For this review, take the finished solid that the model builds, in its own axes (mm). Coordinates: 2 decimals unless noted, no trailing zeros. Write each loop counter-clockwise with the first axis right and the second up, starting at its lowest first coordinate (ties: lowest second). Pieces come first, ordered by that corner, then holes.
1) Mouldability with a two-part tool opening along Y and no side actions: class faces 1 (the face through (1.972, -0.717, 4.943)), 2 (the face through (2.028, -0.09, -3.024)), 3 (the face through (4, 0, 2)) as pulls with the +Y half, pulls with the -Y half, needs draft (parallel to the pull), parting line crosses it, or undercut.
2) To check wall thickness, follow line 1 along Z through (x, y) = (0.85, 4.75); line 2 along Z through (x, y) = (2.9, 0) (3 decimals); line 3 along Y through (x, z) = (1.7, 0) (3 decimals). State the ranges of each line that lie inside material, in increasing order.
3) Insertion check: P1, Ø6, axis at y = -3.5, z = -3, coming from the -X side; P2, Ø1, axis at x = 2.5, y = 4, coming from the +Z side. Each pin has a flat end and moves straight along its axis. Give the tip position at first contact, or say it passes through.
4) We need section D-D on z = -4.5. Write out the cut boundary in (x, y).
5) We need section A-A on z = 0. Write out the cut boundary in (x, y) (3 decimals), then the cut area to 3 significant figures.
6) We need section B-B on y = -1.5. Write out the cut boundary in (x, z) (3 decimals).
7) We need section C-C on z = 4. Write out the cut boundary in (x, y).
from build123d import *

# Parameters (mm, degrees)
BASPROSKE_W         = 4
BASPROSKE_H         = 6
TOOTHCUT_DEPTH      = 10.38083152
TEETHCUTS_COUNT     = 10
TEETHCUTS_ANGLE     = 324
BORSKE_R            = 3.025
BORE_DEPTH          = 50.0000508
BOSS_EXTRUDE1_DEPTH = 4


with BuildPart() as part:
    # BasProSke → Base-Revolve (revolve)
    with BuildSketch(Plane(origin=(0, 0, 0), x_dir=(1, 0, 0), z_dir=(0, 1, 0)), mode=Mode.PRIVATE) as base_revolve_sk:
        with Locations((2, 3)):
            Rectangle(BASPROSKE_W, BASPROSKE_H)
    revolve(base_revolve_sk.sketch.rotate(Axis((-10, 0, 0), (1, 0, 0)), 180), axis=Axis((-10, 0, 0), (1, 0, 0)))

    # TooCutSke → ToothCut (cut, through all)
    with BuildSketch(Plane(origin=(0, 0, 0), x_dir=(0, 0, -1), z_dir=(1, 0, 0))):
        with BuildLine():
            ThreePointArc((0.59278292, 3.701838653), (0, 3.749), (-0.59278292, 3.701838653))
            ThreePointArc((-0.59278292, 3.701838653), (-0.846593509, 4.924114224), (-1.775771316, 5.757784417))
            ThreePointArc((-1.775771316, 5.757784417), (0, 6.0254), (1.775771316, 5.757784417))
            ThreePointArc((1.775771316, 5.757784417), (0.846593509, 4.924114224), (0.59278292, 3.701838653))
        make_face()
    toothcut = extrude(amount=TOOTHCUT_DEPTH, mode=Mode.SUBTRACT)

    # TeethCuts: ToothCut ×10 about axis
    teethcuts_axis = Axis((-10, 0, 0), (1, 0, 0))
    for i in range(1, TEETHCUTS_COUNT):
        add(toothcut.rotate(teethcuts_axis, i * TEETHCUTS_ANGLE / (TEETHCUTS_COUNT - 1)), mode=Mode.SUBTRACT)

    # BorSke → Bore (cut, symmetric)
    with BuildSketch(Plane(origin=(0, 0, 0), x_dir=(0, 0, -1), z_dir=(1, 0, 0))):
        with Locations(Location((0, 0, 0), (0, 0, 180))):
            Circle(BORSKE_R)
    extrude(amount=BORE_DEPTH, both=True, mode=Mode.SUBTRACT)

    # Sketch1 → Boss-Extrude1 (add)
    with BuildSketch(Plane.ZY):
        with BuildLine():
            ThreePointArc((1.565, -2.588706241), (3.025, 0), (1.565, 2.588706241))
            Line((1.565, 2.588706241), (1.565, -2.588706241))
        make_face()
    extrude(amount=-BOSS_EXTRUDE1_DEPTH)


solid = part.part
Result:
1. face 1: undercut
1. face 2: undercut
1. face 3: needs draft
2. line 1: z = -2.22 to -0.76, 0.76 to 2.22
2. line 2: z = -6 to -3.025, 1.565 to 6
2. line 3: y = -3.749 to -3.025, 3.025 to 3.749
3. P1: stops at x = 0
3. P2: stops at z = 4.87
4. outline: (0, -3.66) - (4, -3.66) - (4, -2.42) - (0, -2.42) - close; (0, -0.76) - (4, -0.76) - (4, 0.76) - (0, 0.76) - close; (0, 2.42) - (4, 2.42) - (4, 3.66) - (0, 3.66) - close
5. outline: (0, -3.749) - (4, -3.749) - (4, -3.025) - (0, -3.025) - close; (0, 3.025) - (4, 3.025) - (4, 3.749) - (0, 3.749) - close
5. area: 5.79 mm2
6. outline: (0, -3.436) - (4, -3.436) - (4, -2.627) - (0, -2.627) - close; (0, 1.565) - (4, 1.565) - (4, 3.436) - (0, 3.436) - close
7. outline: (0, -3.62) - (4, -3.62) - (4, -1.97) - (0, -1.97) - close; (0, -0.69) - (4, -0.69) - (4, 0.69) - (0, 0.69) - close; (0, 1.97) - (4, 1.97) - (4, 3.62) - (0, 3.62) - close
